Work out the finished part from the listing and answer in its coordinate system (mm). A direction names the side the tool comes from. Round coordinates to 2 decimals unless told otherwise and drop trailing zeros. Write each loop counter-clockwise with the first axis right and the second up, starting at its lowest first coordinate (ties: lowest second). Pieces come first, ordered by that corner, then holes. Notation, with made-up numbers: (67, 22.5) -> (103, 22.5) arc R17 ccw to (103, 32.5) -> close; hole circle Ø3 at (82, -39.5). An arc over 180 degrees is marked (long way). One line per item, written item: value.
```python
from build123d import *

# Parameters (mm, degrees)
SKETCH_1_R               = 18
EXTRUDE_1_DEPTH          = 10
CUT_EXTRUDE_1_DEPTH      = 28.349588662
PATTERN_CIRCULAR_1_COUNT = 16
SKETCH_3_R               = 12
CUT_EXTRUDE_2_DEPTH      = 4
CUT_EXTRUDE_2_DRAFT      = -6
CUT_EXTRUDE_START        = -10
SKETCH_3_2_R             = 12
CUT_EXTRUDE_3_DEPTH      = 4
CUT_EXTRUDE_3_TAPER      = 6
SKETCH_5_R               = 5
EXTRUDE_2_DEPTH          = 30
CHAMFER_1_SIZE           = 1


with BuildPart() as part:
    # Эскиз1 → Бобышка-Вытянуть1 (new body)
    with BuildSketch(Plane.XY):
        Circle(SKETCH_1_R)
    extrude(amount=-EXTRUDE_1_DEPTH)

    # Эскиз2 → Вырез-Вытянуть1 (cut, through all)
    with BuildSketch(Plane.XY):
        with BuildLine():
            ThreePointArc((3.125667198, 17.726539554), (0, 18), (-3.125667198, 17.726539554))
            ThreePointArc((-3.125667198, 17.726539554), (-1.955189123, 15.973239081), (-1.463398486, 13.923306535))
            ThreePointArc((-1.463398486, 13.923306535), (0, 14), (1.463398486, 13.923306535))
            ThreePointArc((1.463398486, 13.923306535), (1.955189123, 15.973239081), (3.125667198, 17.726539554))
        make_face()
    cut_extrude_1 = extrude(amount=-CUT_EXTRUDE_1_DEPTH, mode=Mode.SUBTRACT)

    # Круговой массив1: Вырез-Вытянуть1 ×16 about axis
    pattern_circular_1_axis = Axis((0, 0, 0), (0, 0, 1))
    for i in range(1, PATTERN_CIRCULAR_1_COUNT):
        add(cut_extrude_1.rotate(pattern_circular_1_axis, i * 360 / PATTERN_CIRCULAR_1_COUNT), mode=Mode.SUBTRACT)


with BuildPart() as cut_extrude_2_tool:
    # Эскиз3 → Вырез-Вытянуть2 (with draft: the straight prism first)
    with BuildSketch(Plane.XY):
        Circle(SKETCH_3_R)
    extrude(amount=-CUT_EXTRUDE_2_DEPTH)
    # Вырез-Вытянуть2: the draft: its side faces are tilted about the plane it starts from
    cut_extrude_2_sides = [cut_extrude_2_tool.faces().sort_by_distance(p)[0] for p in [
        (-12, 0, -2),
    ]]
    draft(cut_extrude_2_sides, Plane.XY, CUT_EXTRUDE_2_DRAFT)


with BuildPart() as part_1:
    add(part.part)

    # Вырез-Вытянуть2: cut by cut_extrude_2_tool
    add(cut_extrude_2_tool.part, mode=Mode.SUBTRACT)

    # Эскиз3<2> → Вырез-Вытянуть3 (cut)
    with BuildSketch(Plane.XY.offset(CUT_EXTRUDE_START)):
        Circle(SKETCH_3_2_R)
    extrude(amount=CUT_EXTRUDE_3_DEPTH, taper=CUT_EXTRUDE_3_TAPER, mode=Mode.SUBTRACT)

    # Эскиз5 → Бобышка-Вытянуть2 (add)
    with BuildSketch(Plane.XY.offset(-4)):
        Circle(SKETCH_5_R)
    extrude(amount=EXTRUDE_2_DEPTH)

    # Фаска1
    chamfer_1_edges = [part_1.edges().sort_by_distance(p)[0] for p in [
        (-5, 0, 26),
    ]]
    chamfer(chamfer_1_edges, length=CHAMFER_1_SIZE)


solid = part_1.part
```
(1) For a pull along Y with two mould halves and no side action, classify faces 6 (the face through (-12.7, 9.92, -4.93)), 7 (the face through (13.99, -7.9, -4.93)), 8 (the face through (-3, 12, -10)) as pulls with the +Y half, pulls with the -Y half, needs draft (parallel to the pull), parting line crosses it, or undercut.
Reported:
face 6: pulls with the +Y half
face 7: undercut
face 8: needs draft
(2) A tool of negligible diameter and unlimited length cuts with its end or side. For faces 1 (the face through (0, 0, 26)), 2 (the face through (9.9, 9.9, -4.9)), 3 (the face through (-9.92, -12.7, -4.93)), 4 (the face through (-7.94, 14.03, -4.93)), 5 (the face through (9.9, -12.65, -4.93)), from which of +Z, -Z, +X, -X, +Y, -Y can it reach the whole face along a straight path? Write none if from no direction.
Reported:
face 1: +Z, +X, -X, +Y, -Y
face 2: +Z, -Z
face 3: +Z, -Z, -X
face 4: +Z, -Z, +Y
face 5: +Z, -Z, +X
(3) Find section A-A on y = 0. Give the vertices of the cut face in (x, z).
Reported:
outline: (-14, -10) -> (-12, -10) -> (-11.58, -6) -> (11.58, -6) -> (12, -10) -> (14, -10) -> (14, 0) -> (12, 0) -> (11.58, -4) -> (5, -4) -> (5, 25) -> (4, 26) -> (-4, 26) -> (-5, 25) -> (-5, -4) -> (-11.58, -4) -> (-12, 0) -> (-14, 0) -> close
(4) Find section C-C on z = 8.5. Give the vertices of the cut face in (x, y), plus the area to 3 significant figures.
Reported:
outline: circle Ø10 at (0, 0)
area: 78.5 mm2
(5) Flat-ended cylindrical pins translate along their axes: pin 1 Ø3 at (x, y) = (-5.5, 12) entering from +Z; pin 2 Ø6 at (y, z) = (-6, 6.5) entering from +X; pin 3 Ø5 at (x, z) = (-5, 13.5) entering from -Y. Find the tip coordinate at first contact, or state that the pin passes through.
Reported:
pin 1: stops at z = 0
pin 2: stops at x = 4
pin 3: stops at y = -4.33
(6) Consider probe 1 along Z at (x, y) = (12, 2.5); probe 2 along Z at (x, y) = (1, 10); probe 3 along Y at (x, z) = (-2, -3.5). Determine where each line is inside the solid, lowest interval first.
Reported:
probe 1: z = -10 to 0
probe 2: z = -6 to -4
probe 3: y = -16.07 to -11.46, -4.58 to 4.58, 11.46 to 16.07
